For this review, take the finished solid that the model builds, in its own axes (mm). A direction names the side the tool comes from. Coordinates: 2 decimals unless noted, no trailing zeros. Loops run counter-clockwise (first coordinate to the right, second up) from the corner with the lowest first, then second, coordinate; pieces in that order, holes last. Notation, with made-up numbers: M -17.75,89 L 37.25,89 A29 ccw 37.25,117 Z; hole C -13.5,56 d8. An arc over 180 degrees is marked long. Use one line per item in the form item = value.
```python
from build123d import *

# Parameters (mm, degrees)
F0_R     = 10.95
F1_DEPTH = 7.2


with BuildPart() as f1:
    # F0 (on Front) → F1 (new body)
    with BuildSketch(Plane.XZ):
        with BuildLine():
            Line((-3.975838, 15.756117), (-3.845241, 15.015463))
            ThreePointArc((-3.845241, 15.015463), (-10.960155, 10.960155), (-15.015463, 3.845241))
            ThreePointArc((-15.015463, 3.845241), (-15.26452, 2.691547), (-15.425069, 1.522246))
            ThreePointArc((-15.425069, 1.522246), (-15.5, 0), (-15.425069, -1.522246))
            ThreePointArc((-15.425069, -1.522246), (-15.26452, -2.691547), (-15.015463, -3.845241))
            ThreePointArc((-15.015463, -3.845241), (-10.960155, -10.960155), (-3.845241, -15.015463))
            ThreePointArc((-3.845241, -15.015463), (-2.691547, -15.26452), (-1.522246, -15.425069))
            ThreePointArc((-1.522246, -15.425069), (0, -15.5), (1.522246, -15.425069))
            ThreePointArc((1.522246, -15.425069), (2.691547, -15.26452), (3.845241, -15.015463))
            ThreePointArc((3.845241, -15.015463), (10.960155, -10.960155), (15.015463, -3.845241))
            ThreePointArc((15.015463, -3.845241), (15.26452, -2.691547), (15.425069, -1.522246))
            ThreePointArc((15.425069, -1.522246), (15.5, 0), (15.425069, 1.522246))
            ThreePointArc((15.425069, 1.522246), (15.26452, 2.691547), (15.015463, 3.845241))
            ThreePointArc((15.015463, 3.845241), (10.960155, 10.960155), (3.845241, 15.015463))
            Line((3.845241, 15.015463), (3.975838, 15.756117))
            ThreePointArc((3.975838, 15.756117), (3.342727, 18.957549), (1.652844, 16.165723))
            Line((1.652844, 16.165723), (1.522246, 15.425069))
            ThreePointArc((1.522246, 15.425069), (0, 15.5), (-1.522246, 15.425069))
            Line((-1.522246, 15.425069), (-1.652844, 16.165723))
            ThreePointArc((-1.652844, 16.165723), (-3.342727, 18.957549), (-3.975838, 15.756117))
        make_face()
        Circle(F0_R, mode=Mode.SUBTRACT)
        with BuildLine():
            ThreePointArc((-15.425069, 1.522246), (-15.26452, 2.691547), (-15.015463, 3.845241))
            Line((-15.015463, 3.845241), (-15.756117, 3.975838))
            ThreePointArc((-15.756117, 3.975838), (-18.957549, 3.342727), (-16.165723, 1.652844))
            Line((-16.165723, 1.652844), (-15.425069, 1.522246))
        make_face()
        with BuildLine():
            ThreePointArc((-15.015463, -3.845241), (-15.26452, -2.691547), (-15.425069, -1.522246))
            Line((-15.425069, -1.522246), (-16.165723, -1.652844))
            ThreePointArc((-16.165723, -1.652844), (-18.957549, -3.342727), (-15.756117, -3.975838))
            Line((-15.756117, -3.975838), (-15.015463, -3.845241))
        make_face()
        with BuildLine():
            ThreePointArc((-1.522246, -15.425069), (-2.691547, -15.26452), (-3.845241, -15.015463))
            Line((-3.845241, -15.015463), (-3.975838, -15.756117))
            ThreePointArc((-3.975838, -15.756117), (-3.342727, -18.957549), (-1.652844, -16.165723))
            Line((-1.652844, -16.165723), (-1.522246, -15.425069))
        make_face()
        with BuildLine():
            ThreePointArc((3.845241, -15.015463), (2.691547, -15.26452), (1.522246, -15.425069))
            Line((1.522246, -15.425069), (1.652844, -16.165723))
            ThreePointArc((1.652844, -16.165723), (3.342727, -18.957549), (3.975838, -15.756117))
            Line((3.975838, -15.756117), (3.845241, -15.015463))
        make_face()
        with BuildLine():
            Line((15.756117, 3.975838), (15.015463, 3.845241))
            ThreePointArc((15.015463, 3.845241), (15.26452, 2.691547), (15.425069, 1.522246))
            Line((15.425069, 1.522246), (16.165723, 1.652844))
            ThreePointArc((16.165723, 1.652844), (18.957549, 3.342727), (15.756117, 3.975838))
        make_face()
        with BuildLine():
            ThreePointArc((15.425069, -1.522246), (15.26452, -2.691547), (15.015463, -3.845241))
            Line((15.015463, -3.845241), (15.756117, -3.975838))
            ThreePointArc((15.756117, -3.975838), (18.957549, -3.342727), (16.165723, -1.652844))
            Line((16.165723, -1.652844), (15.425069, -1.522246))
        make_face()
    extrude(amount=F1_DEPTH)


solid = f1.part
```
1. Consider section A-A on x = 0. Write out the cut boundary in (y, z).
Computed values:
outline = M -7.2,-15.5 L 0,-15.5 L 0,-10.95 L -7.2,-10.95 Z; M -7.2,10.95 L 0,10.95 L 0,15.5 L -7.2,15.5 Z
2. Tool access review of faces 1 (the face through (-15.5, -3.5, 0)), 2 (the face through (8, -7.2, -8)): name each direction out of +Z, -Z, +X, -X, +Y, -Y from which nothing blocks a thin tool from reaching the whole face with its end or side.
Computed values:
face_1 = +Y, -Y
face_2 = +Z, -Z, +X, -X, -Y
3. Draft analysis for pull direction X (two halves, no side actions). For faces 3 (the face through (8, 0, -8)), 4 (the face through (0, -3.5, 15.5)), state which applies: +X half, -X half, draft (parallel to the pull), parting line (faces both ways), or undercut.
Computed values:
face_3 = draft
face_4 = undercut
4. For pin 1 Ø1.5 at (x, z) = (-14, -7) entering from -Y; pin 2 Ø1.5 at (y, z) = (-1, 8.5) entering from +X, all flat-tipped, find the tip position at first contact; note any pin that passes through.
Computed values:
pin_1 = -7.2
pin_2 = 13.42
5. Consider section D-D on x = 11.5. Write out the cut boundary in (y, z).
Computed values:
outline = M -7.2,-10.39 L 0,-10.39 L 0,10.39 L -7.2,10.39 Z
6. Consider section B-B on z = 0. Write out the cut boundary in (x, y), plus the area to 3 significant figures.
Computed values:
outline = M -15.5,-7.2 L -10.95,-7.2 L -10.95,0 L -15.5,0 Z; M 10.95,-7.2 L 15.5,-7.2 L 15.5,0 L 10.95,0 Z
area = 65.5 mm2
7. Wall thickness on line 1 along Z through (x, y) = (0, -2); line 2 along Z through (x, y) = (-7, -5.5); line 3 along X through (y, z) = (-0.5, 10): over which ranges is each line inside the solid? List them lowest first. Write a range as from..to.
Computed values:
line_1 = -15.5..-10.95, 10.95..15.5
line_2 = -13.83..-8.42, 8.42..13.83
line_3 = -11.84..-4.46, 4.46..11.84
